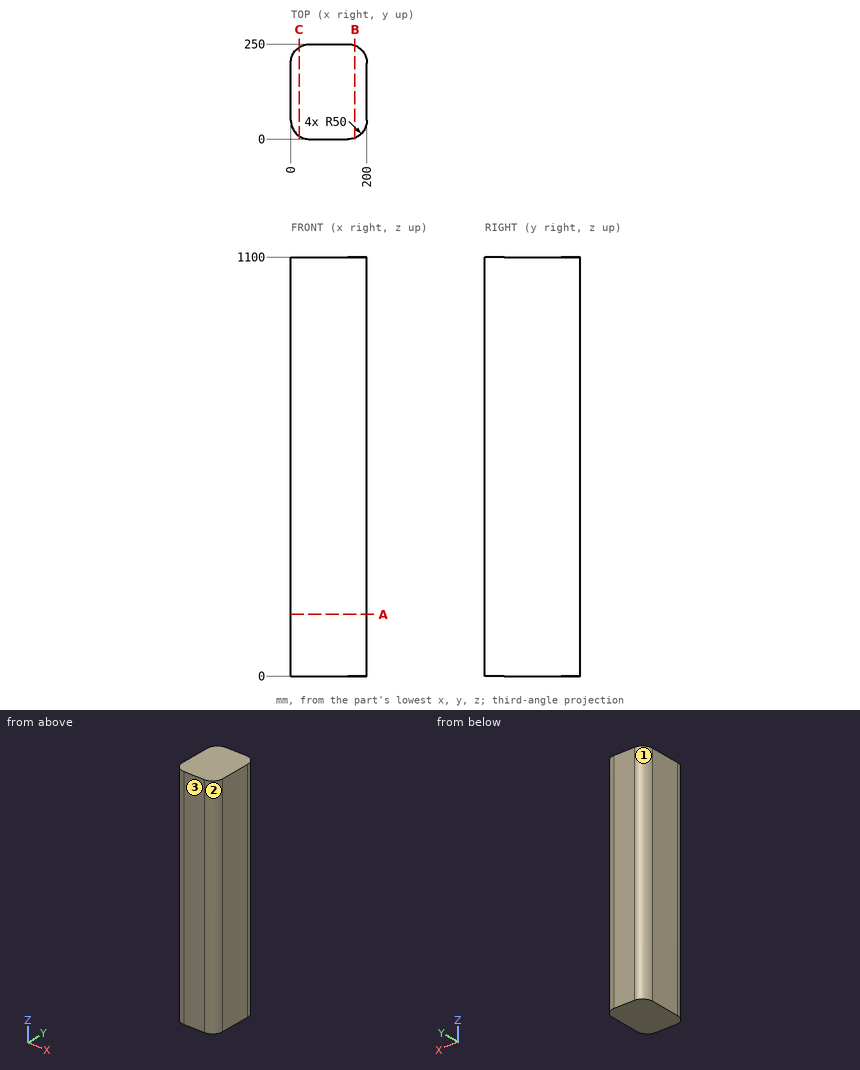
Study the drawing (mm; zero at the part's minimum x, y, z) and answer. Give positions to 0.01 mm unless a question says otherwise; leave off trailing zeros. Order: outer loops, then holes, each group sorted by start corner. A loop starts at its lowest first (then second) coordinate and runs counter-clockwise, first axis right, second up. Notation, with made-up numbers: (21.5, 18.5) -> (65.5, 18.5) arc R34 ccw to (65.5, 54.5) -> close; hole circle Ø3 at (-3, 41.25). An arc over 180 degrees is marked (long way). Put each result on its own line as item: value.
Item 1: Straight lines are drawn through the part: line 1 (X direction, y = 33.5, z = 1029.5); line 2 (X direction, y = 16, z = 816.5); line 3 (Y direction, x = 41.5, z = 375). For each, find the intervals that lie inside material, in ascending order.
Established:
line 1: x = 2.8 to 197.2
line 2: x = 13.34 to 186.66
line 3: y = 0.73 to 249.27
Item 2: A cutting plane is placed at B-B on x = 168. Give the vertices of the cut face in (y, z).
Established:
outline: (3.35, 0) -> (246.65, 0) -> (246.65, 1100) -> (3.35, 1100) -> close
Item 3: A cutting plane is placed at A-A on z = 162. Give the vertices of the cut face in (x, y).
Established:
outline: (0, 50) arc R50 ccw to (50, 0) -> (150, 0) arc R50 ccw to (200, 50) -> (200, 200) arc R50 ccw to (150, 250) -> (50, 250) arc R50 ccw to (0, 200) -> close
Item 4: Given P1, Ø10, axis at x = 165, z = 267.5, coming from the -Y side; P2, Ø12, axis at y = 34, z = 441.5, coming from the +X side; P3, Ø10, axis at x = 167, z = 895.5, coming from the +Y side, each flat-ended and moving along its own axis, determine where each tip first touches the part or whether it passes through.
Established:
P1: stops at y = 1.01
P2: stops at x = 198.99
P3: stops at y = 248.54
Item 5: For a pull along X with two mould halves and no side action, classify the marked faces 1, 2 and 3 as released by +X, released by -X, zero draft, split by the parting line, or undercut.
Established:
face 1: released by -X
face 2: released by +X
face 3: zero draft
Item 6: A cutting plane is placed at C-C on x = 21.5. Give the vertices of the cut face in (y, z).
Established:
outline: (8.92, 0) -> (241.08, 0) -> (241.08, 1100) -> (8.92, 1100) -> close
